```python
from build123d import *

# Parameters (mm, degrees)
PATTERN_CIRCULAR_1_COUNT = 8


with BuildPart() as part:
    # Эскиз1 → Повернуть1 (revolve)
    with BuildSketch(Plane.XY, mode=Mode.PRIVATE) as revolve_1_sk:
        Polygon((-42, 0), (-60, 0), (-60, 9), (-61.5, 9), (-62.5, 10), (-62.5, 28), (-61.5, 29), (-57, 29), (-57, 37), (-60, 40), (-60, 67), (-57, 70), (-46.5, 70), (-46.5, 35), (-31.5, 35), (-31.5, 10), (-42, 10), align=None)
    revolve(revolve_1_sk.sketch.rotate(Axis((0, 0, 0), (0, 1, 0)), 270), axis=Axis((0, 0, 0), (0, 1, 0)))

    # Эскиз5 → Вырез-Повернуть1 (revolve, cut)
    with BuildSketch(Plane.XY):
        Polygon((-43, 0), (-46, 0), (-46, 30), (-50, 30), (-50, 70), (-43, 70), align=None)
    cut_revolve_1 = revolve(axis=Axis((-43, 84.512066433, 0), (0, -1, 0)), mode=Mode.SUBTRACT)

    # Круговой массив1: Вырез-Повернуть1 ×8 about axis, 1 skipped
    pattern_circular_1_axis = Axis((0, 0, 0), (0, -1, 0))
    add([cut_revolve_1.rotate(pattern_circular_1_axis, i * 360 / PATTERN_CIRCULAR_1_COUNT) for i in range(1, PATTERN_CIRCULAR_1_COUNT) if i not in (7,)], mode=Mode.SUBTRACT)


solid = part.part
```
Input: part model. Units: mm. Frame: model coordinates. A direction names the side the tool comes from. Round coordinates to 2 decimals unless told otherwise and drop trailing zeros. Loops run counter-clockwise (first coordinate to the right, second up) from the corner with the lowest first, then second, coordinate; pieces in that order, holes last. Notation, with made-up numbers: (-37.75, 42) -> (-21.75, 42) arc R11 cw to (-21.75, 51) -> close; hole circle Ø5 at (67.25, 16.5). An arc over 180 degrees is marked (long way). One line per item, written item: value.
(1) Material intervals for line 1 (Z direction, x = 0.5, y = 47.5); line 2 (Y direction, x = 48, z = -32.5); line 3 (X direction, y = 54.5, z = -30), sorted ascending. Write a range as [from, to].
Geometry check:
line 1: [-60, -49.98], [49.98, 60]
line 2: [0, 29], [37.97, 69.03]
line 3: [-51.96, -37.39], [37.39, 51.96]
(2) Section B-B (z = 0). Give the number of separate pieces and of enclosed holes in the cut face, plus the area to 3 significant figures.
Geometry check:
separate pieces: 4
enclosed holes: 0
area: 2,060 mm2
(3) Mould query, pull axis Z, two halves, no side actions, for faces 1 (the face through (17.9, 29, -54.4)), 2 (the face through (-2.64, 4.56, 59.94)), 3 (the face through (38.73, 4.93, 16.25)). Classes: pulls with the +Z half, pulls with the -Z half, needs draft (parallel to the pull), parting line crosses it, or undercut.
Geometry check:
face 1: needs draft
face 2: parting line crosses it
face 3: undercut
(4) Pin query (flat end, axial travel): pin 1 (1.5 mm diameter, centred on x = -27.5, y = 53, fed in from +Z); pin 2 (10 mm diameter, centred on y = 52, z = -49.5, fed in from -X); pin 3 (10 mm diameter, centred on y = 20.5, z = -7, fed in from -X); pin 4 (15.5 mm diameter, centred on x = 0.5, z = 45.5, fed in from +Y). Return the tip coordinate at first contact, or that it passes through.
Geometry check:
pin 1: z = 53.71
pin 2: x = -40.25
pin 3: x = -62.47
pin 4: y = 70
(5) Set-up query: faces 4 (the face through (55.645, 33.056, 12.356)), 5 (the face through (33.082, 50.28, -36.874)), 6 (the face through (59, 9, 13)), 7 (the face through (33.18, 15.21, 31.55)). Return all of +Z, -Z, +X, -X, +Y, -Y with unobstructed straight access to the full face (end or side cutting, diameter ignored); none if empty.
Geometry check:
face 4: none
face 5: +Y
face 6: -Y
face 7: +Y, -Y
(6) Section A-A (y = 44). Return the cut outline in (x, z), plus the area to 3 significant figures.
Geometry check:
outline: circle Ø120 at (0, 0); hole (-46.07, -6.29) arc R46.5 ccw to (-37.03, -28.13) arc R7 ccw to (-28.13, -37.03) arc R46.5 ccw to (-6.29, -46.07) arc R7 ccw to (6.29, -46.07) arc R46.5 ccw to (28.13, -37.03) arc R7 ccw to (37.03, -28.13) arc R46.5 ccw to (46.07, -6.29) arc R7 ccw to (46.07, 6.29) arc R46.5 ccw to (37.03, 28.13) arc R7 ccw to (28.13, 37.03) arc R46.5 ccw to (6.29, 46.07) arc R7 ccw to (-6.29, 46.07) arc R46.5 ccw to (-46.07, 6.29) arc R7 ccw to start
area: 4,290 mm2
